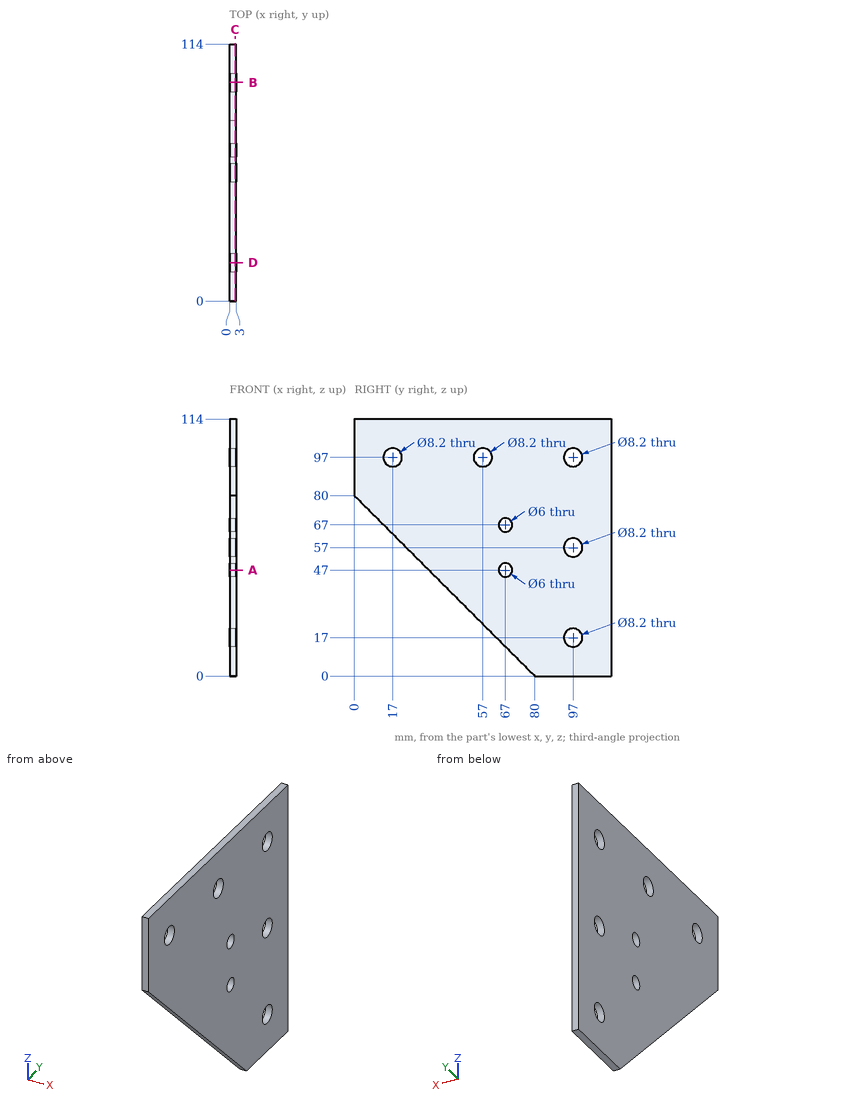
Verification items for this drawing (mm, ordinates from the low corner). Give positions to 0.01 mm unless a question says otherwise; leave off trailing zeros. Loops run counter-clockwise (first coordinate to the right, second up) from the corner with the lowest first, then second, coordinate; pieces in that order, holes last. Notation, with made-up numbers: M 78.25,64.25 L 104.25,64.25 A23 ccw 104.25,94.25 Z; hole C 63,38 d11. An arc over 180 degrees is marked long. Write item = value, one per line.
(1) Sectioned sample at C-C, the plane x = 2.4. Record the cut outline in (y, z).
Answer below:
outline = M 0,80 L 80,0 L 114,0 L 114,114 L 0,114 Z; hole C 17,97 d8.2; hole C 57,97 d8.2; hole C 67,47 d6; hole C 67,67 d6; hole C 97,17 d8.2; hole C 97,57 d8.2; hole C 97,97 d8.2
(2) Gauge pin test, flat end, axial feed: pin 1 Ø7.5 at (y, z) = (97, 57) entering from +X. Record the tip position at first contact, or that the pin passes through.
Answer below:
pin_1 = through
(3) Sectioned sample at D-D, the plane y = 17. Record the cut outline in (x, z).
Answer below:
outline = M 0,63 L 3,63 L 3,92.9 L 0,92.9 Z; M 0,101.1 L 3,101.1 L 3,114 L 0,114 Z
(4) Sectioned sample at A-A, the plane z = 47. Record the cut outline in (x, y).
Answer below:
outline = M 0,33 L 3,33 L 3,64 L 0,64 Z; M 0,70 L 3,70 L 3,114 L 0,114 Z
(5) Material ranges on line 1 (Y direction, x = 1.8, z = 97); line 2 (Z direction, x = 2.7, y = 18.5), recorded low to high. Write a range as [from, to].
Answer below:
line_1 = [0, 12.9], [21.1, 52.9], [61.1, 92.9], [101.1, 114]
line_2 = [61.5, 93.18], [100.82, 114]
(6) Sectioned sample at B-B, the plane y = 97. Record the cut outline in (x, z), plus the area to 3 significant figures.
Answer below:
outline = M 0,0 L 3,0 L 3,12.9 L 0,12.9 Z; M 0,21.1 L 3,21.1 L 3,52.9 L 0,52.9 Z; M 0,61.1 L 3,61.1 L 3,92.9 L 0,92.9 Z; M 0,101.1 L 3,101.1 L 3,114 L 0,114 Z
area = 268 mm2
